Geometry: final body of the model. Coordinates: model frame, mm. A direction names the side the tool comes from. Give positions to 0.01 mm unless a question says otherwise; leave off trailing zeros. Order: outer loops, then holes, each group sorted by start corner. A loop starts at its lowest first (then second) coordinate and runs counter-clockwise, first axis right, second up. Notation, with made-up numbers: (49, 69) - (92, 69) arc R4 cw to (92, 75) - close; hole circle Ø1 at (-5, -15). An arc over 180 degrees is marked (long way). Use one line per item in the form item = value.
from build123d import *

# Parameters (mm, degrees)
BOSS_EXTRUDE1_DEPTH     = 6
FILLET1_R               = 2
CUT_EXTRUDE1_DEPTH      = 95.683683917
CUT_EXTRUDE1_DEPTH_BACK = 95.683683917
SKETCH2_W               = 6
SKETCH2_H               = 20
SKETCH3_W               = 10
SKETCH3_H               = 8
CUT_EXTRUDE2_DEPTH      = 95.683683917
FILLET2_R               = 1
SKETCH4_W               = 20
SKETCH4_H               = 6
CUT_EXTRUDE3_DEPTH      = 95.683683917


with BuildPart() as part:
    # Sketch1 → Boss-Extrude1 (new body)
    with BuildSketch(Plane(origin=(0, 0, 0), x_dir=(1, 0, 0), z_dir=(0, 1, 0))):
        Polygon((65, 20), (65, -20), (73, -20), (73, -60), (-73, -60), (-73, -20), (-65, -20), (-65, 20), (-73, 20), (-73, 60), (73, 60), (73, 20), align=None)
    extrude(amount=BOSS_EXTRUDE1_DEPTH)

    # Fillet1
    fillet1_edges = [part.edges().sort_by_distance(p)[0] for p in [
        (65, 3, 20),
        (73, 3, 20),
        (73, 3, 60),
        (-73, 3, 60),
        (-73, 3, 20),
        (-65, 3, 20),
        (-65, 3, -20),
        (-73, 3, -20),
        (-73, 3, -60),
        (73, 3, -60),
        (73, 3, -20),
        (65, 3, -20),
    ]]
    fillet(fillet1_edges, radius=FILLET1_R)

    # Sketch2 → Cut-Extrude1 (cut, two sides: drawn at the far end of the back side and taken through both)
    with BuildSketch(Plane(origin=(0, 6, 0), x_dir=(1, 0, 0), z_dir=(0, 1, 0)).offset(-CUT_EXTRUDE1_DEPTH_BACK)):
        with Locations((53, 0)):
            Rectangle(SKETCH2_W, SKETCH2_H)
        with Locations((-53, 0)):
            Rectangle(SKETCH2_W, SKETCH2_H)
    extrude(amount=CUT_EXTRUDE1_DEPTH + CUT_EXTRUDE1_DEPTH_BACK, mode=Mode.SUBTRACT)

    # Sketch3 → Cut-Extrude2 (cut, through all)
    with BuildSketch(Plane(origin=(0, 6, 0), x_dir=(1, 0, 0), z_dir=(0, 1, 0))):
        with Locations((0, 4)):
            Rectangle(SKETCH3_W, SKETCH3_H)
        with Locations((0, -12)):
            Rectangle(SKETCH3_W, SKETCH3_H)
    extrude(amount=-CUT_EXTRUDE2_DEPTH, mode=Mode.SUBTRACT)

    # Fillet2
    fillet2_edges = [part.edges().sort_by_distance(p)[0] for p in [
        (5, 3, -8),
        (5, 3, 0),
        (-5, 3, 0),
        (-5, 3, -8),
        (-5, 3, 16),
        (-5, 3, 8),
        (5, 3, 8),
        (5, 3, 16),
    ]]
    fillet(fillet2_edges, radius=FILLET2_R)

    # Sketch4 → Cut-Extrude3 (cut, through all)
    with BuildSketch(Plane(origin=(0, 6, 0), x_dir=(1, 0, 0), z_dir=(0, 1, 0))):
        with Locations((0, 57)):
            Rectangle(SKETCH4_W, SKETCH4_H)
    extrude(amount=-CUT_EXTRUDE3_DEPTH, mode=Mode.SUBTRACT)


solid = part.part
(1) Cut plane B-B on y = 3.55. Give the number of separate pieces and of enclosed holes in the cut face, plus the area to 3 significant figures.
Computed values:
separate_pieces = 1
enclosed_holes = 4
area = 16,400 mm²
(2) Cut plane A-A on x = 52.5. Output: boundary loops of the cut face in (y, z).
Computed values:
outline = (0, -60) - (6, -60) - (6, -10) - (0, -10) - close; (0, 10) - (6, 10) - (6, 60) - (0, 60) - close
(3) Contact query for a flat-ended pin moving along its axis: pin 1 Ø3 at (y, z) = (2, 3) entering from +X. Output: stop coordinate, or through.
Computed values:
pin_1 = 65
(4) Reachability of faces 1 (the face through (69, 3, -20)), 2 (the face through (0, 3, 16)), 3 (the face through (-65, 3, 0)) from +Z, -Z, +X, -X, +Y, -Y: full face, straight path, thin tool, end or side. Return the list, or none.
Computed values:
face_1 = +X, +Y, -Y
face_2 = +Y, -Y
face_3 = -X, +Y, -Y
(5) Ray query, line 1 along Z through (x, y) = (1, 3.2); line 2 along X through (y, z) = (3.3, -2); line 3 along Z through (x, y) = (50.5, 3.25). Return the intervals inside material, ascending.
Computed values:
line_1 = -54 to -8, 0 to 8, 16 to 60
line_2 = -65 to -56, -50 to -5, 5 to 50, 56 to 65
line_3 = -60 to -10, 10 to 60
(6) Pull-direction query (Z, two-part tool) for faces 4 (the face through (1, 3, 60)), 5 (the face through (53, 3, -10)), 6 (the face through (73, 3, -40)), 7 (the face through (40, 3, -60)); classes: released by +Z, released by -Z, zero draft, split by the parting line, or undercut.
Computed values:
face_4 = released by +Z
face_5 = undercut
face_6 = zero draft
face_7 = released by -Z
